Read the model definition and answer for the solid it produces. Units are mm, in the model's axes. Face numbers are marked on the shaded views. A direction names the side the tool comes from. Coordinates: 2 decimals unless noted, no trailing zeros. Write each loop counter-clockwise with the first axis right and the second up, starting at its lowest first coordinate (ties: lowest second). Pieces come first, ordered by that corner, then holes. Notation, with made-up numbers: (54, 35.25) -> (112, 35.25) arc R24 cw to (112, 72.25) -> close; hole circle Ø9 at (85.5, 22). An arc over 180 degrees is marked (long way). One line per item, written item: value. Start each with the question number.
Autodesk Inventor part; units mm, degrees
ref_plane "YZ Plane" through (0, 0, 0) normal (1, 0, 0) x (0, 1, 0)
ref_plane "XZ Plane" through (0, 0, 0) normal (0, 1, 0) x (-1, 0, 0)
ref_plane "XY Plane" through (0, 0, 0) normal (0, 0, 1) x (1, 0, 0)
sketch "Sketch1" plane through (0, 0, 0) normal (0, 1, 0) x (-1, 0, 0)
  line L0 (0, 0) -> (40.64, 0)
  line L1 (40.64, 0) -> (40.64, 67.945)
  line L2 (40.64, 67.945) -> (0, 67.945)
  line L3 (0, 67.945) -> (0, 0)
  line L4 (10.16, 0) -> (10.16, 67.945)
  line L5 (30.48, 0) -> (30.48, 67.945)
  dimension "d0" = 40.64
  dimension "d1" = 67.945
extrude "Extrusion1" add sketch "Sketch1" along normal blind 5.08
sketch "Sketch2" plane through (0, 5.08, 0) normal (0, 1, 0) x (1, 0, 0)
  line L0 (0, 0) -> (-40.64, 0)
  line L1 (-40.64, -67.945) -> (0, -67.945)
  line L2 (0, -67.945) -> (0, 0)
  line L3 (-10.16, 0) -> (-10.16, -67.945)
  line L4 (-30.48, 0) -> (-30.48, -67.945)
extrude "Extrusion2" add sketch "Sketch2" along normal blind 20.32 contours L3 L1 L4 L0
sketch "Sketch3" plane through (0, 25.4, 0) normal (0, 1, 0) x (1, 0, 0)
  line L0 (-30.48, -67.945) -> (-10.16, -67.945)
  line L1 (-10.16, -67.945) -> (-10.16, 0)
  line L2 (-25.4, -55.88) -> (-15.24, -55.88)
  line L3 (-25.4, -55.88) -> (-25.4, -67.945)
  line L4 (-15.24, -55.88) -> (-15.24, -67.945)
  point P0 (0, 0)
extrude "Extrusion3" add sketch "Sketch3" along normal blind 52.705
sketch "Sketch4" plane through (-15.24, 25.4, 67.945) normal (1, 0, 0) x (0, 0, -1)
  circle A0 centre (6.0325, 8.89) radius 2.2225
  circle A1 centre (6.0325, 43.815) radius 2.2225
  point P0 (67.945, -25.4)
  dimension "d8" = 4.445
  dimension "d10" = 4.445
extrude "Extrusion4" cut sketch "Sketch4" against normal blind 52.705
sketch "Sketch5" plane through (0, 5.08, 0) normal (0, 1, 0) x (1, 0, 0)
  circle A0 centre (-5.08, -12.7) radius 2.2225
  circle A1 centre (-5.08, -55.245) radius 2.2225
  dimension "d14" = 4.445
  dimension "d16" = 4.445
extrude "Extrusion5" cut sketch "Sketch5" against normal blind 52.705
sketch "Sketch6" plane through (0, 5.08, 0) normal (0, 1, 0) x (1, 0, 0)
  circle A0 centre (-35.56, -12.7) radius 2.2225
  circle A1 centre (-35.56, -55.245) radius 2.2225
  point P0 (0, 0)
  dimension "d21" = 4.445
  dimension "d22" = 4.445
extrude "Extrusion6" cut sketch "Sketch6" against normal blind 52.705
fillet "Fillet1" radius 3.175 1 edges at (-40.64, 2.54, 0)
fillet "Fillet2" radius 3.175 1 edges at (-40.64, 2.54, 67.945)
fillet "Fillet3" radius 3.175 1 edges at (0, 2.54, 0)
fillet "Fillet4" radius 3.175 1 edges at (0, 2.54, 67.945)
fillet "Fillet7" radius 3.175 1 edges at (-10.16, 15.24, 67.945)
fillet "Fillet8" radius 3.175 1 edges at (-30.48, 15.24, 67.945)
fillet "Fillet9" radius 3.175 1 edges at (-10.16, 15.24, 0)
fillet "Fillet10" radius 3.175 1 edges at (-30.48, 15.24, 0)
properties part number "Autonomous - Encoder Mount"
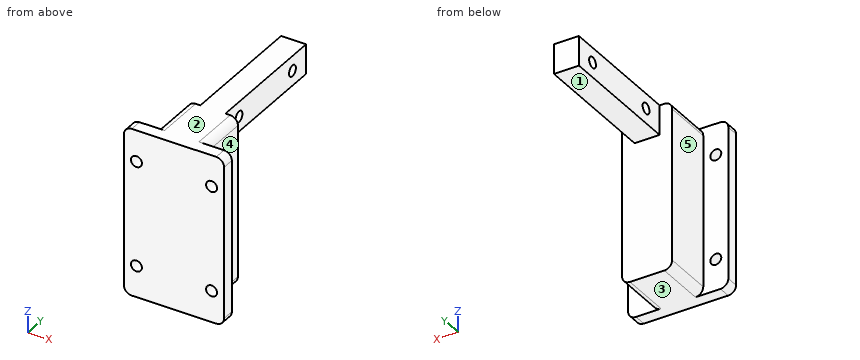
1. Given pin 1 (5 mm diameter, centred on x = -35.56, z = 55.245, fed in from +Y); pin 2 (10 mm diameter, centred on y = 10.5, z = 46.5, fed in from -X); pin 3 (12 mm diameter, centred on x = -27, z = 43.5, fed in from +Y), each flat-ended and moving along its own axis, determine where each tip first touches the part or whether it passes through.
2. Find the intervals of material crossed by probe 1 along Z at (x, y) = (-5, 1) (3 decimals); probe 2 along Z at (x, y) = (-19, 34) (3 decimals); probe 3 along Y at (x, z) = (-33, 37), in increasing order. Write a range as from..to.
3. A cutting plane is placed at B-B on z = 12.7. Give the vertices of the cut face in (x, y), then the cut area to 3 significant figures.
4. A tool of negligible diameter and unlimited length cuts with its end or side. For the marked faces 1, 2, 3, 4 and 5, from which of +Z, -Z, +X, -X, +Y, -Y can it reach the whole face along a straight path? Write none if from no direction.
5. A cutting plane is placed at A-A on y = 34.29. Give the vertices of the cut face in (x, z) (3 decimals).
6. A cutting plane is placed at D-D on z = 50.5. Give the vertices of the cut face in (x, y), then the cut area to 3 significant figures.
7. A cutting plane is placed at C-C on x = -5.08. Give the vertices of the cut face in (y, z) (1 decimal).
Derived:
1. pin 1: stops at y = 5.08
1. pin 2: stops at x = -30.48
1. pin 3: stops at y = 25.4
2. probe 1: z = 0..10.479, 14.921..53.024, 57.466..67.945
2. probe 2: z = 55.88..59.709, 64.116..67.945
2. probe 3: y = 0..5.08
3. outline: (-40.64, 0) -> (-37.78, 0) -> (-37.78, 5.08) -> (-40.64, 5.08) -> close; (-33.34, 0) -> (-7.3, 0) -> (-7.3, 5.08) -> (-10.16, 5.08) -> (-10.16, 25.4) -> (-30.48, 25.4) -> (-30.48, 5.08) -> (-33.34, 5.08) -> close; (-2.86, 0) -> (0, 0) -> (0, 5.08) -> (-2.86, 5.08) -> close
3. area: 574 mm2
4. face 1: -Z, +X, -X, +Y
4. face 2: +Z, +X, -X, +Y, -Y
4. face 3: -Z, +X, -X, +Y, -Y
4. face 4: +Z, -Z, +X, +Y
4. face 5: +Z, -Z, -X, +Y
5. outline: (-25.4, 55.88) -> (-15.24, 55.88) -> (-15.24, 59.69) -> (-25.4, 59.69) -> close; (-25.4, 64.135) -> (-15.24, 64.135) -> (-15.24, 67.945) -> (-25.4, 67.945) -> close
6. outline: (-40.64, 0) -> (0, 0) -> (0, 5.08) -> (-10.16, 5.08) -> (-10.16, 25.4) -> (-30.48, 25.4) -> (-30.48, 5.08) -> (-40.64, 5.08) -> close
6. area: 619 mm2
7. outline: (0, 0) -> (5.1, 0) -> (5.1, 10.5) -> (0, 10.5) -> close; (0, 14.9) -> (5.1, 14.9) -> (5.1, 53) -> (0, 53) -> close; (0, 57.5) -> (5.1, 57.5) -> (5.1, 67.9) -> (0, 67.9) -> close
